Could you check a few things on this model? Use its own coordinates, in mm. Round coordinates to 2 decimals unless told otherwise and drop trailing zeros. Loops run counter-clockwise (first coordinate to the right, second up) from the corner with the lowest first, then second, coordinate; pieces in that order, holes last. Notation, with made-up numbers: M 6,4.5 L 24,4.5 A25 cw 24,16.5 Z; hole C 89.5,8 d1. An arc over 180 degrees is marked long. Answer in a Markdown table with one row per item.
```python
from build123d import *

# Parameters (mm, degrees)
F0_R     = 2.4
F1_DEPTH = 3.2


with BuildPart() as f1:
    # F0 (on Top) → F1 (new body)
    with BuildSketch(Plane.XY):
        with BuildLine():
            ThreePointArc((0, 12.175), (-3.725, 15.9), (-7.45, 12.175))
            Line((-7.45, 12.175), (-7.45, -7.45))
            Line((-7.45, -7.45), (12.175, -7.45))
            ThreePointArc((12.175, -7.45), (15.9, -3.725), (12.175, 0))
            Line((12.175, 0), (0, 0))
            Line((0, 0), (0, 12.175))
        make_face()
        Polygon((-4.725, -2.725), (-4.725, -1.225), (-2.725, -1.225), (-2.725, -2.725), (-1.225, -2.725), (-1.225, -4.725), (-2.725, -4.725), (-2.725, -6.225), (-4.725, -6.225), (-4.725, -4.725), (-6.225, -4.725), (-6.225, -2.725), align=None, mode=Mode.SUBTRACT)
        with Locations((4.225, -3.725)):
            Circle(F0_R, mode=Mode.SUBTRACT)
        Polygon((11.175, -2.725), (11.175, -1.225), (13.175, -1.225), (13.175, -2.725), (14.675, -2.725), (14.675, -4.725), (13.175, -4.725), (13.175, -6.225), (11.175, -6.225), (11.175, -4.725), (9.675, -4.725), (9.675, -2.725), align=None, mode=Mode.SUBTRACT)
        with Locations((-3.725, 4.225)):
            Circle(F0_R, mode=Mode.SUBTRACT)
        Polygon((-4.725, 13.175), (-4.725, 14.675), (-2.725, 14.675), (-2.725, 13.175), (-1.225, 13.175), (-1.225, 11.175), (-2.725, 11.175), (-2.725, 9.675), (-4.725, 9.675), (-4.725, 11.175), (-6.225, 11.175), (-6.225, 13.175), align=None, mode=Mode.SUBTRACT)
    extrude(amount=F1_DEPTH)


solid = f1.part
```
1) I want a section at B-B, the plane y = 2.25. Please give me the cut outline in (x, z).
Computed:
| item | result |
|---|---|
| outline | M -7.45,0 L -5.09,0 L -5.09,3.2 L -7.45,3.2 Z; M -2.36,0 L 0,0 L 0,3.2 L -2.36,3.2 Z |
2) I need wall thicknesses on line 1 (Y direction, x = 12, z = 2.4) (3 decimals); line 2 (X direction, y = 12.25, z = 2.25) (3 decimals). Which ranges of each line are inside material? Lowest first, please.
Computed:
| item | result |
|---|---|
| line 1 | y = -7.45 to -6.225, -1.225 to 0 |
| line 2 | x = -7.449 to -6.225, -1.225 to -0.001 |
3) Will these pins go through, and if not, where does the flat tip stop? P1, Ø1, axis at x = 12.5, z = 1, coming from the -Y side; P2, Ø1.2, axis at y = -5.5, z = 1.5, coming from the +X side; P3, Ø0.8, axis at x = 14, z = 2, coming from the -Y side; P4, Ø0.8, axis at y = 13.5, z = 1.5, coming from the -X side.
Computed:
| item | result |
|---|---|
| P1 | stops at y = -7.45 |
| P2 | stops at x = 15.71 |
| P3 | stops at y = -7.17 |
| P4 | stops at x = -7.33 |
4) I want a section at A-A, the plane x = -2. Please give me the cut outline in (y, z) (3 decimals), plus the area to 3 significant figures.
Computed:
| item | result |
|---|---|
| outline | M -7.45,0 L -4.725,0 L -4.725,3.2 L -7.45,3.2 Z; M -2.725,0 L 2.556,0 L 2.556,3.2 L -2.725,3.2 Z; M 5.894,0 L 11.175,0 L 11.175,3.2 L 5.894,3.2 Z; M 13.175,0 L 15.477,0 L 15.477,3.2 L 13.175,3.2 Z |
| area | 49.9 mm² |
5) If we mould it in two halves opening along Y, with no side actions, what happens to faces 1 (the face through (-3.64, 15.9, 1.58)), 2 (the face through (2, -7.45, 2)), 3 (the face through (14.675, -4, 2))? For each: released by +Y, released by -Y, zero draft, split by the parting line, or undercut.
Computed:
| item | result |
|---|---|
| face 1 | released by +Y |
| face 2 | released by -Y |
| face 3 | undercut |
6) I want a section at C-C, the plane x = 2.5. Please give me the cut outline in (y, z), plus the area to 3 significant figures.
Computed:
| item | result |
|---|---|
| outline | M -7.45,0 L -5.39,0 L -5.39,3.2 L -7.45,3.2 Z; M -2.06,0 L 0,0 L 0,3.2 L -2.06,3.2 Z |
| area | 13.2 mm² |
7) I want a section at D-D, the plane z = 1.15. State how many separate pieces and enclosed holes the cut face has, plus the area to 3 significant figures.
Computed:
| item | result |
|---|---|
| separate pieces | 1 |
| enclosed holes | 5 |
| area | 196 mm² |
